Autodesk Inventor part; units mm, degrees
ref_plane "YZ Plane" through (0, 0, 0) normal (1, 0, 0) x (0, 1, 0)
ref_plane "XZ Plane" through (0, 0, 0) normal (0, 1, 0) x (-1, 0, 0)
ref_plane "XY Plane" through (0, 0, 0) normal (0, 0, 1) x (1, 0, 0)
sketch "Sketch1" plane through (0, 0, 0) normal (0, 0, 1) x (1, 0, 0)
  line L0 (0, 6.4) -> (0, -4.8)
  line L1 (-12, 0) -> (16, 0)
  line L2 (-10, 4) -> (10, 4)
  line L3 (10, 4) -> (10, -4)
  line L4 (10, -4) -> (-10, -4)
  line L5 (-10, -4) -> (-10, 4)
  dimension "d0" = 20
  dimension "d1" = 8
extrude "Extrusion1" add sketch "Sketch1" along normal blind 9
shell "Shell1" thickness 0.5 removed faces 1 at (3.3333, -1.3333, 9)
sketch "Sketch2" plane through (-10, -4, 0) normal (0, -1, 0) x (1, 0, 0)
  line L0 (20, 9) -> (0, 9) construction
  line L1 (19.5, 0.5) -> (0.5, 0.5) construction
  line L2 (10, 11.7) -> (10, -0.9) construction
  line L3 (7.5, 9) -> (12.5, 9)
  line L4 (12.5, 9) -> (12.5, 0.5)
  line L5 (12.5, 0.5) -> (7.5, 0.5)
  line L6 (7.5, 0.5) -> (7.5, 9)
  dimension "d5" = 5
extrude "Extrusion2" cut sketch "Sketch2" against normal up to next
properties part number "config - c9g5 connector"
CAD build for the part. Positions are in the model's coordinates, mm. A direction names the side the tool comes from. Round coordinates to 2 decimals unless told otherwise and drop trailing zeros. Loops run counter-clockwise (first coordinate to the right, second up) from the corner with the lowest first, then second, coordinate; pieces in that order, holes last. Notation, with made-up numbers: (33.25, 77) - (59.25, 77) arc R6 cw to (59.25, 86) - close; hole circle Ø7 at (61, 63.25). An arc over 180 degrees is marked (long way). Put each result on its own line as item: value.
1. Slice it at B-B on y = -1.75. List the corners of the cut face in (x, z).
Geometry check:
outline: (-10, 0) - (10, 0) - (10, 9) - (9.5, 9) - (9.5, 0.5) - (-9.5, 0.5) - (-9.5, 9) - (-10, 9) - close
2. Pin check, flat tip, straight feed: P1, Ø2.5, axis at x = 0.5, z = 4.5, coming from the -Y side. Stop position of the tip, or through.
Geometry check:
P1: y = 3.5
3. Slice it at C-C on z = 6. List the corners of the cut face in (x, y), and give its area (3 significant figures).
Geometry check:
outline: (-10, -4) - (-2.5, -4) - (-2.5, -3.5) - (-9.5, -3.5) - (-9.5, 3.5) - (9.5, 3.5) - (9.5, -3.5) - (2.5, -3.5) - (2.5, -4) - (10, -4) - (10, 4) - (-10, 4) - close
area: 24.5 mm²
4. Slice it at A-A on x = 6.75. List the corners of the cut face in (y, z).
Geometry check:
outline: (-4, 0) - (4, 0) - (4, 9) - (3.5, 9) - (3.5, 0.5) - (-3.5, 0.5) - (-3.5, 9) - (-4, 9) - close
5. 3-axis set-ups, long thin cutter, end or side, ignore diameter. For faces 1 (the flat face through (5, -4, 4)), 2 (the flat face through (-9.5, 0, 5)): which of +Z, -Z, +X, -X, +Y, -Y reach the whole face in a straight line?
Geometry check:
face 1: +Z, -Z, +X, -X, -Y
face 2: +Z
6. Wall check: line 1 (X direction, y = -1.5, z = 2.25); line 2 (Y direction, x = 2.75, z = 8); line 3 (Z direction, x = -1.75, y = 2.5). Give the ranges that are in metal, low to high.
Geometry check:
line 1: -10 to -9.5, 9.5 to 10
line 2: -4 to -3.5, 3.5 to 4
line 3: 0 to 0.5
7. Two-plate mould, pull along X, no slides. Class faces 3 (the flat face through (10, 0, 4)), 4 (the flat face through (0, 0, 0.5)), 5 (the flat face through (0, 4, 4)): released by +X, released by -X, zero draft, split by the parting line, or undercut.
Geometry check:
face 3: released by +X
face 4: undercut
face 5: zero draft
